Part model, mm, in its own coordinate system. A direction names the side the tool comes from. Give positions to 0.01 mm unless a question says otherwise; leave off trailing zeros. Order: outer loops, then holes, each group sorted by start corner. A loop starts at its lowest first (then second) coordinate and runs counter-clockwise, first axis right, second up. Notation, with made-up numbers: M 53,77 L 71,77 A34 cw 71,116 Z; hole C -7,50.25 d11. An arc over 180 degrees is marked long. Return JSON: item names as keys, results as strings.
from build123d import *

# Parameters (mm, degrees)
SKETCH_1_R          = 1.95
EXTRUDE_1_DEPTH     = 19
SKETCH_4_W          = 2
SKETCH_4_H          = 9
EXTRUDE_2_DEPTH     = 1.95
CUT_EXTRUDE_1_DEPTH = 21.359396
EXTRUDE_4_DEPTH     = 15.9
SKETCH_9_R          = 2
CUT_EXTRUDE_2_DEPTH = 17


with BuildPart() as part:
    # 스케치1 → 보스-돌출1 (new body)
    with BuildSketch(Plane.XY):
        Circle(SKETCH_1_R)
    extrude(amount=EXTRUDE_1_DEPTH)

    # 스케치4 → 보스-돌출2 (add, symmetric)
    with BuildSketch(Plane(origin=(0, 0, 0), x_dir=(0, 0, -1), z_dir=(1, 0, 0))):
        with Locations((-1, -2.55)):
            Rectangle(SKETCH_4_W, SKETCH_4_H)
    extrude(amount=EXTRUDE_2_DEPTH, both=True)

    # 스케치5 → 컷-돌출1 (cut, through all)
    with BuildSketch(Plane.XY.offset(19)):
        with BuildLine():
            Line((-1.95, 1.95), (-1.95, 0))
            ThreePointArc((-1.95, 0), (-1.378858, 1.378858), (0, 1.95))
            Line((0, 1.95), (-1.95, 1.95))
        make_face()
        with BuildLine():
            ThreePointArc((0, 1.95), (1.378858, 1.378858), (1.95, 0))
            Line((1.95, 0), (1.95, 1.95))
            Line((1.95, 1.95), (0, 1.95))
        make_face()
    extrude(amount=-CUT_EXTRUDE_1_DEPTH, mode=Mode.SUBTRACT)

    # 스케치8 → 보스-돌출4 (add)
    with BuildSketch(Plane.XY.offset(2)):
        with BuildLine():
            ThreePointArc((1.95, -2.279803), (0, -3), (-1.95, -2.279803))
            Line((-1.95, -2.279803), (-1.95, -7.05))
            Line((-1.95, -7.05), (1.95, -7.05))
            Line((1.95, -7.05), (1.95, -2.279803))
        make_face()
    extrude(amount=EXTRUDE_4_DEPTH)

    # 스케치9 → 컷-돌출2 (cut)
    with BuildSketch(Plane.ZY.offset(1.95)):
        with Locations((9, -7.55)):
            Circle(SKETCH_9_R)
    extrude(amount=-CUT_EXTRUDE_2_DEPTH, mode=Mode.SUBTRACT)


solid = part.part
Q1. 3-axis set-ups, long thin cutter, end or side, ignore diameter. For faces 5 (the flat face through (0, -5, 17.9)), 6 (the flat face through (0, -7.05, 14)), 7 (the cylindrical face through (0, -3, 10)): which of +Z, -Z, +X, -X, +Y, -Y reach the whole face in a straight line?
Established:
{"face 5": "+Z, +X, -X, -Y", "face 6": "+Z, -Z, +X, -X, -Y", "face 7": "+Z"}
Q2. Band-saw the part on C-C (y = -1.5). Give the cut face in (x, z), then the cut area to 3 significant figures.
Established:
{"outline": "M -1.95,0 L 1.95,0 L 1.95,2 L 1.25,2 L 1.25,19 L -1.25,19 L -1.25,2 L -1.95,2 Z", "area": "50.2 mm²"}
Q3. Band-saw the part on B-B (x = -1.6). Give the cut face in (y, z), then the cut area to 3 significant figures.
Established:
{"outline": "M -7.05,0 L 1.11,0 L 1.11,19 L -1.11,19 L -1.11,2 L -2.54,2 L -2.54,17.9 L -7.05,17.9 L -7.05,10.94 A2 cw -7.05,7.06 Z", "area": "122 mm²"}
Q4. Band-saw the part on A-A (z = 3.5). Give the cut face in (x, y), then the cut area to 3 significant figures.
Established:
{"outline": "M -1.95,-7.05 L 1.95,-7.05 L 1.95,-2.28 A3 cw -1.95,-2.28 Z; C 0,0 d3.9", "area": "28.6 mm²"}
Q5. Pin check, flat tips, straight feed: pin 1 (1.5 mm diameter, centred on x = -1, z = 2, fed in from +Y); pin 2 (1.2 mm diameter, centred on x = 0, y = -3.5, fed in from +Z); pin 3 (1.5 mm diameter, centred on x = 1.5, z = 5, fed in from +Y). Stop position of each tip, or through.
Established:
{"pin 1": "stops at y = 1.93", "pin 2": "stops at z = 17.9", "pin 3": "stops at y = 1.8"}
Q6. Band-saw the part on D-D (z = 8). Give the cut face in (x, y).
Established:
{"outline": "M -1.95,-5.82 L 1.95,-5.82 L 1.95,-2.28 A3 cw -1.95,-2.28 Z; C 0,0 d3.9"}
Q7. Probe line 1 along Z through (x, y) = (-1.7, -4.5); line 2 along Y through (x, z) = (1.4, 13); line 3 along Y through (x, z) = (-1.15, 14.5). List the from-to ranges inside material, lowest first.
Established:
{"line 1": "z = 0 to 17.9", "line 2": "y = -7.05 to -2.65, -1.36 to 1.36", "line 3": "y = -7.05 to -2.77, -1.57 to 1.57"}
Q8. Two-plate mould, pull along X, no slides. Class faces 1 (the flat face through (0, -2.2, 2)), 2 (the flat face through (0, -3, 0)), 3 (the flat face through (1.95, -4, 9)), 4 (the flat face through (-1.95, -4, 9)): +X half, -X half, draft (parallel to the pull), parting line (faces both ways), or undercut.
Established:
{"face 1": "undercut", "face 2": "draft", "face 3": "+X half", "face 4": "-X half"}
